```python
from build123d import *

# Parameters (mm, degrees)
ESQUISSE1_W                   = 44.2
ESQUISSE1_H                   = 52.2
BOSS_EXTRU_1_DEPTH            = 52.2
ENL_V_MAT_EXTRU_2_DEPTH       = 74.209903702
ENL_V_MAT_EXTRU_2_DEPTH_BACK  = 44.2
ENL_V_MAT_EXTRU_3_DEPTH       = 74.209903702
ENL_V_MAT_EXTRU_3_DEPTH_BACK  = 44.2
ENL_V_MAT_EXTRU_4_DEPTH       = 78.059003368
ENL_V_MAT_EXTRU_4_DEPTH_BACK  = 46
ENL_V_MAT_EXTRU_5_DEPTH       = 78.059003368
ENL_V_MAT_EXTRU_5_DEPTH_BACK  = 46
ENL_V_MAT_EXTRU_7_DEPTH       = 45.550224466
ENL_V_MAT_EXTRU_7_DEPTH_BACK  = 45.550224466
ENL_V_MAT_EXTRU_8_DEPTH       = 78.059003368
ENL_V_MAT_EXTRU_8_DEPTH_BACK  = 46
ENL_V_MAT_EXTRU_9_DEPTH       = 75.993733072
ENL_V_MAT_EXTRU_9_DEPTH_BACK  = 46
ESQUISSE13_R                  = 3
BOSS_EXTRU_2_DEPTH            = 21
ENL_V_MAT_EXTRU_10_DEPTH      = 84.625713749
ENL_V_MAT_EXTRU_10_DEPTH_BACK = 49
ENL_V_MAT_EXTRU_11_DEPTH      = 82.074163579
ENL_V_MAT_EXTRU_11_DEPTH_BACK = 49


with BuildPart() as part:
    # Esquisse1 → Boss.-Extru.1 (new body)
    with BuildSketch(Plane.XY):
        Rectangle(ESQUISSE1_W, ESQUISSE1_H)
    extrude(amount=BOSS_EXTRU_1_DEPTH)

    # Esquisse2 → Enlèv. mat.-Extru.2 (cut, two sides: drawn at the far end of the back side and taken through both)
    with BuildSketch(Plane(origin=(22.1, 0, 0), x_dir=(0, 0, -1), z_dir=(1, 0, 0)).offset(-ENL_V_MAT_EXTRU_2_DEPTH_BACK)):
        Polygon((-201.352290675, -19.9), (-52.2, -19.9), (-28.55, -19.9), (-28.55, -21.45), (-32.25, -21.45), (-32.25, -22.45), (-28.745559959, -26.1), (74.553898465, -133.690091099), (-39.180744024, -409.461834307), (-315.086933163, -295.671743208), align=None)
    extrude(amount=ENL_V_MAT_EXTRU_2_DEPTH + ENL_V_MAT_EXTRU_2_DEPTH_BACK, mode=Mode.SUBTRACT)

    # Esquisse3 → Enlèv. mat.-Extru.3 (cut, two sides: drawn at the far end of the back side and taken through both)
    with BuildSketch(Plane(origin=(22.1, 0, 0), x_dir=(0, 0, -1), z_dir=(1, 0, 0)).offset(-ENL_V_MAT_EXTRU_3_DEPTH_BACK)):
        Polygon((149.152290675, -19.9), (0, -19.9), (-23.65, -19.9), (-23.65, -21.45), (-19.95, -21.45), (-19.95, -22.45), (-23.454440041, -26.1), (-126.753898465, -133.690091099), (-13.019255976, -409.461834307), (262.886933163, -295.671743208), align=None)
    extrude(amount=ENL_V_MAT_EXTRU_3_DEPTH + ENL_V_MAT_EXTRU_3_DEPTH_BACK, mode=Mode.SUBTRACT)

    # Esquisse4 → Enlèv. mat.-Extru.4 (cut, two sides: drawn at the far end of the back side and taken through both)
    with BuildSketch(Plane(origin=(0, 26.1, 0), x_dir=(1, 0, 0), z_dir=(0, 1, 0)).offset(-ENL_V_MAT_EXTRU_4_DEPTH_BACK)):
        Polygon((-15.9, -191.333109619), (-15.9, -52.2), (-15.9, -28.55), (-17.45, -28.55), (-17.45, -32.25), (-18.45, -32.25), (-22.1, -28.745559959), (-122.462816227, 67.614843274), (-379.791464965, -38.281593439), (-273.228648738, -297.229546332), align=None)
    extrude(amount=ENL_V_MAT_EXTRU_4_DEPTH + ENL_V_MAT_EXTRU_4_DEPTH_BACK, mode=Mode.SUBTRACT)

    # Esquisse5 → Enlèv. mat.-Extru.5 (cut, two sides: drawn at the far end of the back side and taken through both)
    with BuildSketch(Plane(origin=(0, 26.1, 0), x_dir=(1, 0, 0), z_dir=(0, 1, 0)).offset(-ENL_V_MAT_EXTRU_5_DEPTH_BACK)):
        Polygon((-15.9, 139.133109619), (-15.9, 0), (-15.9, -23.65), (-17.45, -23.65), (-17.45, -19.95), (-18.45, -19.95), (-22.1, -23.454440041), (-122.462816228, -119.814843274), (-379.791464965, -13.918406561), (-273.228648738, 245.029546332), align=None)
    extrude(amount=ENL_V_MAT_EXTRU_5_DEPTH + ENL_V_MAT_EXTRU_5_DEPTH_BACK, mode=Mode.SUBTRACT)

    # Esquisse6 → Enlèv. mat.-Extru.7 (cut, two sides: drawn at the far end of the back side and taken through both)
    with BuildSketch(Plane.XY.offset(28.55).offset(-ENL_V_MAT_EXTRU_7_DEPTH_BACK)):
        Polygon((-161.22284167, -19.9), (-22.1, -19.9), (-15.9, -19.9), (-15.9, -26.093649616), (-15.9, -165.216491285), (-212.645110561, -361.97019968), (-357.967952231, -216.653708395), align=None)
    extrude(amount=ENL_V_MAT_EXTRU_7_DEPTH + ENL_V_MAT_EXTRU_7_DEPTH_BACK, mode=Mode.SUBTRACT)

    # Esquisse11 → Enlèv. mat.-Extru.8 (cut, two sides: drawn at the far end of the back side and taken through both)
    with BuildSketch(Plane(origin=(0, 26.1, 0), x_dir=(1, 0, 0), z_dir=(0, 1, 0)).offset(-ENL_V_MAT_EXTRU_8_DEPTH_BACK)):
        Polygon((164.227968273, -49.1), (22.1, -49.1), (-15.9, -49.1), (-158.027968273, -49.1), (-158.027968273, -333.355936546), (164.227968273, -333.355936546), align=None)
    extrude(amount=ENL_V_MAT_EXTRU_8_DEPTH + ENL_V_MAT_EXTRU_8_DEPTH_BACK, mode=Mode.SUBTRACT)

    # Esquisse12 → Enlèv. mat.-Extru.9 (cut, two sides: drawn at the far end of the back side and taken through both)
    with BuildSketch(Plane(origin=(0, 26.1, 0), x_dir=(1, 0, 0), z_dir=(0, 1, 0)).offset(-ENL_V_MAT_EXTRU_9_DEPTH_BACK)):
        Polygon((159.687460199, -3.1), (22.1, -3.1), (-15.9, -3.1), (-153.487460199, -3.1), (-153.487460199, 272.074920398), (159.687460199, 272.074920398), align=None)
    extrude(amount=ENL_V_MAT_EXTRU_9_DEPTH + ENL_V_MAT_EXTRU_9_DEPTH_BACK, mode=Mode.SUBTRACT)

    # Esquisse13 → Boss.-Extru.2 (add)
    with BuildSketch(Plane(origin=(22.1, 0, 0), x_dir=(0, 0, -1), z_dir=(1, 0, 0))):
        with Locations(Location((-27.1, 3.6, 0), (0, 0, 270))):
            Circle(ESQUISSE13_R)
    extrude(amount=BOSS_EXTRU_2_DEPTH)

    # Esquisse15 → Enlèv. mat.-Extru.10 (cut, two sides: drawn at the far end of the back side and taken through both)
    with BuildSketch(Plane(origin=(0, 26.1, 0), x_dir=(1, 0, 0), z_dir=(0, 1, 0)).offset(-ENL_V_MAT_EXTRU_10_DEPTH_BACK)):
        Polygon((-15.9, 114.859960703), (-15.9, -23.65), (-15.9, -28.55), (-15.9, -167.059960703), (-292.919921407, -167.059960703), (-292.919921407, 114.859960703), align=None)
    extrude(amount=ENL_V_MAT_EXTRU_10_DEPTH + ENL_V_MAT_EXTRU_10_DEPTH_BACK, mode=Mode.SUBTRACT)

    # Esquisse16 → Enlèv. mat.-Extru.11 (cut, two sides: drawn at the far end of the back side and taken through both)
    with BuildSketch(Plane.ZY.offset(15.9).offset(-ENL_V_MAT_EXTRU_11_DEPTH_BACK)):
        Polygon((-91.491856556, -19.9), (23.65, -19.9), (28.55, -19.9), (143.691856556, -19.9), (143.691856556, -250.183713112), (-91.491856556, -250.183713112), align=None)
    extrude(amount=ENL_V_MAT_EXTRU_11_DEPTH + ENL_V_MAT_EXTRU_11_DEPTH_BACK, mode=Mode.SUBTRACT)


solid = part.part
```
Can you work these out from the model? Positions are in its coordinate system, mm. A direction names the side the tool comes from. Coordinates: 2 decimals unless noted, no trailing zeros. Loops run counter-clockwise (first coordinate to the right, second up) from the corner with the lowest first, then second, coordinate; pieces in that order, holes last.
1) I need wall thicknesses on probe 1 along X at (y, z) = (-16, 12). Which ranges of the line are inside material? Lowest first, please.
2) Which directions (+Z, -Z, +X, -X, +Y, -Y) give clear straight access to the entire face, cutting with the end or side of a thin tool? Please do faces 1 (the cylindrical face through (32.453, 2.216, 29.762)), 2 (the flat face through (3, -19.9, 26)).
3) Imagine slicing it at D-D on z = 17.5. List the corners of the cut face in (x, y) for me, plus the area to 3 significant figures.
4) For pin 1 (2 mm diameter, centred on y = 11.5, z = 32.5, fed in from +X), with a flat end and sliding along its axis, tell me the tip position at first contact or that it passes through.
5) Imagine slicing it at B-B on z = 27.1. List the corners of the cut face in (x, y) for me, plus the area to 3 significant figures.
6) Imagine slicing it at A-A on y = 3.6. List the corners of the cut face in (x, z) for me.
7) Imagine slicing it at C-C on y = 10. List the corners of the cut face in (x, z) for me.
Completed:
1. probe 1: x = -15.9 to 22.1
2. face 1: +X
2. face 2: +Z, -Z, +X, -X, -Y
3. outline: (-15.9, -19.9) - (22.1, -19.9) - (22.1, 26.1) - (-15.9, 26.1) - close
3. area: 1,750 mm2
4. pin 1: stops at x = 22.1
5. outline: (-15.9, -19.9) - (22.1, -19.9) - (22.1, 0.6) - (43.1, 0.6) - (43.1, 6.6) - (22.1, 6.6) - (22.1, 26.1) - (-15.9, 26.1) - close
5. area: 1,870 mm2
6. outline: (-15.9, 3.1) - (22.1, 3.1) - (22.1, 24.1) - (43.1, 24.1) - (43.1, 30.1) - (22.1, 30.1) - (22.1, 49.1) - (-15.9, 49.1) - close
7. outline: (-15.9, 3.1) - (22.1, 3.1) - (22.1, 49.1) - (-15.9, 49.1) - close
